Build history of the part. All positions in model axes, mm. Face numbers are marked on the shaded views. A direction names the side the tool comes from. Coordinates: 2 decimals unless noted, no trailing zeros. Order: outer loops, then holes, each group sorted by start corner. A loop starts at its lowest first (then second) coordinate and runs counter-clockwise, first axis right, second up. Notation, with made-up numbers: (56, 65.5) - (98, 65.5) arc R34 cw to (98, 95.5) - close; hole circle Ø10 at (86, 87.5). An arc over 180 degrees is marked (long way). Write each question's results on one line, items separated by ' | '. Start each with the question number.
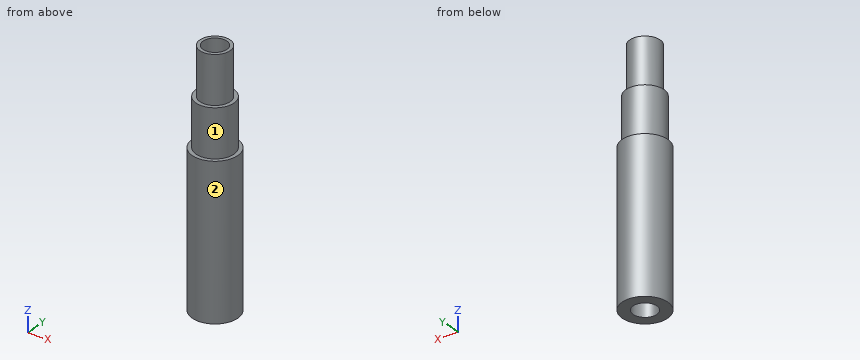
Autodesk Inventor part; units mm, degrees
ref_plane "YZ Plane" through (0, 0, 0) normal (1, 0, 0) x (0, 1, 0)
ref_plane "XZ Plane" through (0, 0, 0) normal (0, 1, 0) x (-1, 0, 0)
ref_plane "XY Plane" through (0, 0, 0) normal (0, 0, 1) x (1, 0, 0)
sketch "Sketch1" plane through (0, 0, 0) normal (0, 0, 1) x (1, 0, 0)
  circle A0 centre (0, 0) radius 4.7625
  dimension "d0" = 9.525
extrude "Extrusion1" add sketch "Sketch1" along normal blind 31.75
sketch "Sketch2" plane through (0, 0, 31.75) normal (0, 0, 1) x (1, 0, 0)
  circle A0 centre (0, 0) radius 4.7625
  circle A1 centre (0, 0) radius 3.9688
  dimension "d4" = 7.9375
extrude "Extrusion2" add sketch "Sketch2" along normal blind 9.9817 contours A1
sketch "Sketch3" plane through (0, 0, 41.7317) normal (0, 0, 1) x (1, 0, 0)
  circle A0 centre (0, 0) radius 3.9687
  circle A1 centre (0, 0) radius 3.175
  dimension "d8" = 6.35
extrude "Extrusion3" add sketch "Sketch3" along normal blind 9.9568 contours A1
sketch "Sketch4" plane through (0, 0, 51.6885) normal (0, 0, 1) x (1, 0, 0)
  circle A0 centre (0, 0) radius 3.175
hole "Hole1" at (0, 0, 51.6885) direction (0, 0, -1) diameter 4.9784 end through all
properties part number "Main Connecting Standoff Stepped"
Item 1: Which spindle directions (+Z, -Z, +X, -X, +Y, -Y) get a long thin tool onto all of the face, cutting with end or side? Do the marked faces 1 and 2. Say none if no direction does.
Item 2: Slice it at C-C (z = 11). Write the cut outline in (x, y) (1 decimal).
Item 3: Probe probe 1 along Y at (x, z) = (0, 32); probe 2 along Y at (x, z) = (0, 26.5); probe 3 along Z at (x, y) = (3.25, -0.25). List the from-to ranges inside material, lowest first.
Item 4: Flat gauge pins, fed straight in: P1, Ø5.5, axis at x = 0, y = 0, coming from the +Z side; P2, Ø3, axis at y = 1.5, z = 37, coming from the -X side; P3, Ø4, axis at x = 0.5, z = 34, coming from the -Y side; P4, Ø2, axis at y = 3.5, z = 45.5, coming from the +X side. Where does each tip first touch, or does it go through?
Item 5: Slice it at D-D (z = 37). Write the cut outline in (x, y).
Resolved:
1) face 1: +Z | face 2: +Z, -Z
2) outline: circle Ø9.5 at (0, 0); hole circle Ø5 at (0, 0)
3) probe 1: -3.97 to -2.49, 2.49 to 3.97 | probe 2: -4.76 to -2.49, 2.49 to 4.76 | probe 3: 0 to 41.73
4) P1: z = 51.69 | P2: x = -3.97 | P3: y = -3.97 | P4: x = 1.96
5) outline: circle Ø7.94 at (0, 0); hole circle Ø4.98 at (0, 0)
